Part model, mm, in its own coordinate system. A direction names the side the tool comes from. Give positions to 0.01 mm unless a question says otherwise; leave off trailing zeros. Order: outer loops, then holes, each group sorted by start corner. A loop starts at its lowest first (then second) coordinate and runs counter-clockwise, first axis right, second up. Notation, with made-up numbers: (60, -14.75) -> (116, -14.75) arc R23 ccw to (116, 17.25) -> close; hole circle Ø9 at (50.25, -33). An arc over 180 degrees is marked (long way). Write item = value, one per line. Start each with the question number.
(1) Probe line 1 along X through (y, z) = (-95.6, -1); line 2 along X through (y, z) = (-85.5, 1.1); line 3 along Z through (x, y) = (41.5, -96.2). List the from-to ranges inside material, lowest first. Write a range as from..to.
(2) Saw through at D-D, the plane y = -78.5. List the corners of the cut face in (x, z), then the cut area to 3 significant figures.
(3) Saw through at A-A, the plane x = 42.25. List the corners of the cut face in (y, z), then the cut area to 3 significant figures.
(4) Flat gauge pins, fed straight in: pin 1 (10 mm diameter, centred on x = 37.5, z = -7.5, fed in from +Y); pin 2 (4.5 mm diameter, centred on y = -82, z = -7.5, fed in from -X); pin 3 (5.5 mm diameter, centred on x = 42.5, y = -85.5, fed in from -Z). Where does each tip first touch, or does it go through?
(5) Saw through at C-C, the plane x = 46. List the corners of the cut face in (y, z), then the cut area to 3 significant figures.
(6) Saw through at B-B, the plane z = -7.5. List the corners of the cut face in (x, y).
(7) Two-plate mould, pull along X, no slides. Class faces 4 (the flat face through (45, -87, 3)), 5 (the flat face through (49, -85, -9)), 6 (the flat face through (52, -87, -6)), 7 (the cylindrical face through (40.51, -95.48, -6.74)): pulls with the +X half, pulls with the -X half, needs draft (parallel to the pull), parting line crosses it, or undercut.
(8) Which spindle directions (+Z, -Z, +X, -X, +Y, -Y) get a long thin tool onto all of the face, cutting with end or side? Do faces 1 (the flat face through (50, -90, -15)), 2 (the flat face through (37.836, -91, 1)), 3 (the flat face through (43, -94, -7)). Say none if no direction does.
Autodesk Inventor part; units mm, degrees
ref_plane "YZ Plane" through (0, 0, 0) normal (1, 0, 0) x (0, 1, 0)
ref_plane "XZ Plane" through (0, 0, 0) normal (0, 1, 0) x (-1, 0, 0)
ref_plane "XY Plane" through (0, 0, 0) normal (0, 0, 1) x (1, 0, 0)
ref_plane "작업 평면1" through (0, 0, 0) normal (0, 0, 1) x (1, 0, 0)
sketch "스케치1" plane through (0, 0, 0) normal (0, 0, 1) x (1, 0, 0)
  line L0 (49, -94) -> (-72, -94) construction
  line L1 (49, -88) -> (49, -94) construction
  line L2 (-72, -88) -> (49, -88) construction
  line L3 (-72, -94) -> (-72, -88) construction
  line L4 (43, 88) -> (43, -88) construction
  line L5 (49, -88) -> (43, -88) construction
  line L6 (49, 88) -> (49, -88) construction
  line L7 (49, 88) -> (43, 88) construction
  line L8 (-72, -88) -> (43, -88) construction
  line L9 (43, -88) -> (43, 88) construction
  line L10 (-72, 88) -> (43, 88) construction
  line L11 (-72, 88) -> (-72, -88) construction
  circle A0 centre (-2.8299, 17.3) radius 1.35 construction
  circle A1 centre (19.1701, -17.3) radius 1.35 construction
  circle A2 centre (-24.8299, 17.3) radius 1.35 construction
  circle A3 centre (19.1701, 17.3) radius 1.35 construction
  circle A4 centre (-2.8299, -17.3) radius 1.35 construction
  circle A5 centre (-24.8299, -17.3) radius 1.35 construction
  arc A6 (-27.4299, -13.5) -> (-26.3299, -14.6) centre (-26.3299, -13.5) ccw construction
  line L12 (-27.4299, -13.5) -> (-27.4299, 13.5) construction
  arc A7 (-26.3299, 14.6) -> (-27.4299, 13.5) centre (-26.3299, 13.5) ccw construction
  line L13 (-26.3299, 14.6) -> (28.6701, 14.6) construction
  line L14 (28.6701, 14.6) -> (28.6701, -14.6) construction
  line L15 (28.6701, -14.6) -> (-26.3299, -14.6) construction
  line L16 (-72, -88) -> (43, -88) construction
  line L17 (43, -88) -> (43, 88) construction
  line L18 (-72, 88) -> (43, 88) construction
  line L19 (-72, 88) -> (-72, -88) construction
  circle A8 centre (-2.8299, 17.3) radius 1.35 construction
  circle A9 centre (19.1701, -17.3) radius 1.35 construction
  circle A10 centre (-24.8299, 17.3) radius 1.35 construction
  circle A11 centre (19.1701, 17.3) radius 1.35 construction
  circle A12 centre (-2.8299, -17.3) radius 1.35 construction
  circle A13 centre (-24.8299, -17.3) radius 1.35 construction
  arc A14 (-27.4299, -13.5) -> (-26.3299, -14.6) centre (-26.3299, -13.5) ccw construction
  line L20 (-27.4299, -13.5) -> (-27.4299, 13.5) construction
  arc A15 (-26.3299, 14.6) -> (-27.4299, 13.5) centre (-26.3299, 13.5) ccw construction
  line L21 (-26.3299, 14.6) -> (28.6701, 14.6) construction
  line L22 (28.6701, 14.6) -> (28.6701, -14.6) construction
  line L23 (28.6701, -14.6) -> (-26.3299, -14.6) construction
  line L24 (43, 88) -> (43, -88)
  line L25 (49, -88) -> (43, -88)
  line L26 (49, 88) -> (49, -88)
  line L27 (49, 88) -> (43, 88)
  line L28 (49, -94) -> (-72, -94)
  line L29 (49, -88) -> (49, -94)
  line L30 (-72, -88) -> (49, -88)
  line L31 (-72, -94) -> (-72, -88)
  line L32 (-72, -88) -> (43, -88)
  line L33 (43, -88) -> (43, 88)
  line L34 (-72, 88) -> (43, 88)
  line L35 (-72, 88) -> (-72, -88)
  circle A16 centre (-2.8299, 17.3) radius 1.35
  circle A17 centre (19.1701, -17.3) radius 1.35
  circle A18 centre (-24.8299, 17.3) radius 1.35
  circle A19 centre (19.1701, 17.3) radius 1.35
  circle A20 centre (-2.8299, -17.3) radius 1.35
  circle A21 centre (-24.8299, -17.3) radius 1.35
  arc A22 (-27.4299, -13.5) -> (-26.3299, -14.6) centre (-26.3299, -13.5) ccw
  line L36 (-27.4299, -13.5) -> (-27.4299, 13.5)
  arc A23 (-26.3299, 14.6) -> (-27.4299, 13.5) centre (-26.3299, 13.5) ccw
  line L37 (-26.3299, 14.6) -> (28.6701, 14.6)
  line L38 (28.6701, 14.6) -> (28.6701, -14.6)
  line L39 (28.6701, -14.6) -> (-26.3299, -14.6)
  line L40 (49, -94) -> (-72, -94)
  line L41 (49, -88) -> (49, -94)
  line L42 (-72, -88) -> (49, -88)
  line L43 (-72, -94) -> (-72, -88)
  line L44 (49, -94) -> (49, -77)
  line L45 (49, -94) -> (32, -94)
  line L46 (49, -77) -> (43, -77)
  line L47 (32, -94) -> (32, -88)
  line L48 (49, -94) -> (32, -94)
  line L49 (32, -94) -> (32, -77)
  line L50 (32, -77) -> (49, -77)
  line L51 (49, -77) -> (49, -94)
  line L52 (49, -94) -> (29, -94)
  line L53 (29, -94) -> (29, -77)
  line L54 (29, -77) -> (49, -77)
  line L55 (49, -77) -> (49, -94)
  point P0 (0, 0)
  dimension "d0" = 17
  dimension "d1" = 17
  dimension "d28" = 20
extrude "돌출1" add sketch "스케치1" along normal blind 3 contours L46 L26 L25 L24 | L24 L30 L49 L50 | L25 L29 L28 L47 L30 | L49 L30 L53 L54 | L47 L28 L53 L30
sketch "스케치2" plane through (49, -94, 0) normal (1, 0, 0) x (0, 0, -1)
  line L0 (40.7085, 16) -> (17.2915, 16)
  arc A0 (16.3174, 17.226) -> (17.2915, 16) centre (17.2915, 17) ccw
  line L1 (16.3174, 17.226) -> (28.0259, 67.6827)
  arc A1 (29.9741, 67.6827) -> (28.0259, 67.6827) centre (29, 67.4566) ccw
  line L2 (29.9741, 67.6827) -> (41.6826, 17.226)
  arc A2 (40.7085, 16) -> (41.6826, 17.226) centre (40.7085, 17) ccw
  line L3 (34.1853, 94.226) -> (45.1259, 141.3733)
  arc A3 (47.1, 141.1472) -> (45.1259, 141.3733) centre (46.1, 141.1472) ccw
  line L4 (47.1, 141.1472) -> (47.1, 46.8528)
  arc A4 (45.1259, 46.6267) -> (47.1, 46.8528) centre (46.1, 46.8528) ccw
  line L5 (45.1259, 46.6267) -> (34.1853, 93.774)
  arc A5 (34.1853, 94.226) -> (34.1853, 93.774) centre (35.1594, 94) ccw
  line L6 (10.9, 46.8528) -> (10.9, 141.1472)
  arc A6 (12.8741, 141.3733) -> (10.9, 141.1472) centre (11.9, 141.1472) ccw
  line L7 (12.8741, 141.3733) -> (23.8147, 94.226)
  arc A7 (23.8147, 93.774) -> (23.8147, 94.226) centre (22.8406, 94) ccw
  line L8 (23.8147, 93.774) -> (12.8741, 46.6267)
  arc A8 (10.9, 46.8528) -> (12.8741, 46.6267) centre (11.9, 46.8528) ccw
  line L9 (28.0259, 120.3173) -> (16.3174, 170.774)
  arc A9 (17.2915, 172) -> (16.3174, 170.774) centre (17.2915, 171) ccw
  line L10 (17.2915, 172) -> (40.7085, 172)
  arc A10 (41.6826, 170.774) -> (40.7085, 172) centre (40.7085, 171) ccw
  line L11 (41.6826, 170.774) -> (29.9741, 120.3173)
  arc A11 (28.0259, 120.3173) -> (29.9741, 120.3173) centre (29, 120.5434) ccw
  line L12 (58, 182) -> (0, 182)
  line L13 (0, 182) -> (0, 6)
  line L14 (58, 6) -> (0, 6)
  line L15 (58, 6) -> (58, 182)
  line L16 (58, 0) -> (0, 0)
  line L17 (58, 6) -> (58, 0)
  line L18 (0, 6) -> (58, 6)
  line L19 (0, 6) -> (0, 0)
  line L20 (6, 182) -> (6, 6)
  line L21 (0, 0) -> (0, 17)
  line L22 (0, 17) -> (-3, 17)
  line L23 (-3, 0) -> (-3, 17)
  line L24 (0, 0) -> (-3, 0)
  line L25 (-3, 0) -> (22, 0)
  line L26 (22, 0) -> (22, 17)
  line L27 (22, 17) -> (-3, 17)
  line L28 (-3, 17) -> (-3, 0)
  point P0 (0, 94)
  point P1 (0, 0)
  point P2 (22, 0)
  point P3 (22, 16)
  point P4 (16.2915, 17)
  point P5 (0, 17)
  dimension "d4" = 25
extrude "돌출2" add sketch "스케치2" along normal blind 3 contours L26 L14 L20 L27 A0 L0 | L0 A0 L27 L26 | L26 L16 L19 L14 | L14 L13 L27 L20 | L19 L24 L23 L22 L13
sketch "스케치3" plane through (32, -94, 0) normal (0, -1, 0) x (1, 0, 0)
  line L0 (20, 3) -> (20, -22)
  line L1 (0, 0) -> (0, 3)
  line L2 (20, -22) -> (0, -22)
  line L3 (0, -22) -> (0, 3)
  line L4 (0, 3) -> (20, 3)
  line L5 (20, 3) -> (20, -22)
  line L6 (20, 3) -> (-3, 3)
  line L7 (-3, 3) -> (-3, -22)
  line L8 (-3, -22) -> (20, -22)
  line L9 (20, -22) -> (20, 3)
  point P0 (-32, 0)
  point P1 (20, 3)
  point P2 (0, -22)
  dimension "d27" = 23
extrude "돌출3" add sketch "스케치3" along normal blind 3
sketch "스케치8" plane through (0, 0, 3) normal (0, 0, 1) x (1, 0, 0)
  line L0 (29, -97) -> (52, -97)
  line L1 (29, -77) -> (52, -77)
  line L2 (52, -97) -> (34, -97)
  line L3 (34, -97) -> (34, -77)
  line L4 (34, -77) -> (52, -77)
  line L5 (52, -77) -> (52, -97)
  line L6 (34, -77) -> (29, -77)
  line L7 (29, -77) -> (29, -97)
  line L8 (29, -97) -> (34, -97)
  line L9 (34, -97) -> (34, -77)
  point P0 (0, 0)
  dimension "d29" = 18
extrude "돌출8" cut sketch "스케치8" against normal blind 50 contours L7 L1 L3 L0
sketch "스케치10" plane through (52, -94, 0) normal (1, 0, 0) x (0, 0, -1)
  line L0 (-3, 17) -> (-3, -3)
  line L1 (22, -3) -> (-3, -3)
  line L2 (-3, 17) -> (17, 17)
  line L3 (17, 17) -> (17, -3)
  line L4 (17, -3) -> (-3, -3)
  line L5 (-3, -3) -> (-3, 17)
  line L6 (-3, 17) -> (15, 17)
  line L7 (15, 17) -> (15, -3)
  line L8 (15, -3) -> (-3, -3)
  line L9 (-3, -3) -> (-3, 17)
  line L10 (15, 17) -> (22, 17)
  line L11 (22, 17) -> (22, -3)
  line L12 (22, -3) -> (15, -3)
  line L13 (15, -3) -> (15, 17)
  point P0 (0, 94)
  point P1 (15, 17)
  point P2 (17, 17)
  dimension "d32" = 20
  dimension "d33" = 18
extrude "돌출9" cut sketch "스케치10" against normal blind 50 contours L2 L3 L1 L7 | L10 L11 L1 L3
sketch "스케치12" plane through (32, -94, 0) normal (0, 1, 0) x (1, 0, 0)
  circle A0 centre (14, 1) radius 1.25
  circle A1 centre (8, 17) radius 1.25
  circle A2 centre (8, 1) radius 1.25
  circle A3 centre (14, 17) radius 1.25
  line L0 (4, -3) -> (20, -3)
  line L1 (20, 21) -> (20, -3)
  line L2 (4, 21) -> (20, 21)
  line L3 (4, 21) -> (4, -3)
  circle A4 centre (14, 1) radius 1.25
  arc A5 (8.2846, 1.2694) -> (7.5179, 0.8668) centre (7.785, 1.2894) ccw
  point P0 (-32, 0)
extrude "돌출10" cut sketch "스케치12" against normal blind 50 contours A0 | A2
sketch "스케치13" plane through (0, 0, 0) normal (0, 0, -1) x (-1, 0, 0)
  line L0 (-34, -94) -> (-34, -77)
  line L1 (-49, -77) -> (-34, -77)
  line L2 (-49, -94) -> (-49, -77)
  line L3 (-46.75, -94) -> (-49, -94)
  line L4 (-45.25, -94) -> (-46.75, -94)
  line L5 (-40.75, -94) -> (-45.25, -94)
  line L6 (-39.25, -94) -> (-40.75, -94)
  line L7 (-34, -94) -> (-39.25, -94)
  line L8 (-41.5, -94) -> (-41.5, -77)
  line L9 (-34, -85.5) -> (-49, -85.5)
  circle A0 centre (-41.5, -85.5) radius 1.25
  point P0 (0, 0)
  dimension "d38" = 2.5
extrude "돌출11" cut sketch "스케치13" against normal blind 50 contours A0 L8 L9 | L9 L8 A0 | L9 A0 L8 | L8 A0 L9
sketch "스케치14" plane through (49, -94, 0) normal (-1, 0, 0) x (0, 0, 1)
  line L0 (-15, 17) -> (-15, 0)
  line L1 (0, 0) -> (-15, 0)
  line L2 (0, 0) -> (0, 17)
  line L3 (-15, 17) -> (0, 17)
  line L4 (-15, 8.5) -> (0, 8.5)
  line L5 (0, 0) -> (-15, 0)
  line L6 (-7.5, 0) -> (-7.5, 17)
  circle A0 centre (-7.5, 8.5) radius 1.25
  point P0 (0, 94)
  dimension "d41" = 2.5
extrude "돌출12" cut sketch "스케치14" against normal blind 50 contours A0 L6 L4 | L4 L6 A0 | A0 L4 L6 | L4 A0 L6
sketch "스케치15" plane through (32, -94, 0) normal (0, 1, 0) x (1, 0, 0)
  arc A0 (8.75, 0) -> (7.25, 0) centre (8, 1) ccw
  line L0 (8.75, 0) -> (13.25, 0)
  arc A1 (14.75, 0) -> (13.25, 0) centre (14, 1) ccw
  line L1 (14.75, 0) -> (17, 0)
  line L2 (17, 0) -> (17, 15)
  line L3 (17, 15) -> (2, 15)
  line L4 (2, 15) -> (2, 0)
  line L5 (2, 0) -> (7.25, 0)
  line L6 (9.5, 15) -> (9.5, 0)
  line L7 (8.75, 0) -> (13.25, 0)
  line L8 (2, 15) -> (2, 0)
  line L9 (2, 7.5) -> (17, 7.5)
  circle A2 centre (9.5, 7.5) radius 1.25
  point P0 (-32, 0)
  dimension "d44" = 2.5
extrude "돌출13" cut sketch "스케치15" against normal blind 50 contours A2 L9 L6 | L6 L9 A2 | L9 A2 L6 | L6 A2 L9
sketch "스케치16" plane through (0, 0, 0) normal (0, 0, -1) x (-1, 0, 0)
  circle A0 centre (-41.5, -85.5) radius 1.25
  line L0 (-34, -94) -> (-34, -77)
  line L1 (-49, -77) -> (-34, -77)
  line L2 (-49, -94) -> (-49, -77)
  line L3 (-46.75, -94) -> (-49, -94)
  line L4 (-45.25, -94) -> (-46.75, -94)
  line L5 (-40.75, -94) -> (-45.25, -94)
  line L6 (-39.25, -94) -> (-40.75, -94)
  line L7 (-34, -94) -> (-39.25, -94)
  point P0 (0, 0)
extrude "돌출14" cut sketch "스케치16" against normal blind 0.5
sketch "스케치17" plane through (34, -77, 3) normal (0, 1, 0) x (1, 0, 0)
  line L0 (18, 0) -> (0, 0)
  line L1 (0, 0) -> (3.8357, 0)
  line L2 (3.8357, 0) -> (3.8357, 17.9453)
  line L3 (3.8357, 17.9453) -> (0, 17.9453)
  line L4 (0, 17.9453) -> (0, 0)
  point P0 (-34, 3)
  point P1 (3.8357, 0)
extrude "돌출15" cut sketch "스케치17" against normal blind 50
properties part number "10" material "LCP 플라스틱"
Results list:
q1.line_1 = 37.84..38.75, 41.25..44.75, 47.25..52
q1.line_2 = 37.84..40.25, 42.75..52
q1.line_3 = -15..-8.75, -6.25..3
q2.outline = (37.84, 0.5) -> (49, 0.5) -> (49, -15) -> (52, -15) -> (52, 3) -> (37.84, 3) -> close
q2.area = 81.9 mm^2
q3.outline = (-97, -15) -> (-94, -15) -> (-94, -8.5) -> (-97, -8.5) -> close; (-97, -6.5) -> (-94, -6.5) -> (-94, 0.5) -> (-86.5, 0.5) -> (-86.5, 3) -> (-97, 3) -> close; (-84.5, 0.5) -> (-77, 0.5) -> (-77, 3) -> (-84.5, 3) -> close
q3.area = 85.5 mm^2
q4.pin_1 = -94
q4.pin_2 = 49
q4.pin_3 = 0.5
q5.outline = (-97, -15) -> (-94, -15) -> (-94, -2.25) -> (-97, -2.25) -> close; (-97, 0.25) -> (-94, 0.25) -> (-94, 0.5) -> (-77, 0.5) -> (-77, 3) -> (-97, 3) -> close
q5.area = 89.0 mm^2
q6.outline = (37.84, -97) -> (40.25, -97) -> (40.25, -94) -> (37.84, -94) -> close; (42.75, -97) -> (52, -97) -> (52, -86.75) -> (49, -86.75) -> (49, -94) -> (42.75, -94) -> close; (49, -84.25) -> (52, -84.25) -> (52, -77) -> (49, -77) -> close
q7.face_4 = needs draft
q7.face_5 = pulls with the -X half
q7.face_6 = pulls with the +X half
q7.face_7 = undercut
q8.face_1 = -Z, +X, -X, +Y, -Y
q8.face_2 = +Z, -X, +Y, -Y
q8.face_3 = -Z, -X, +Y
